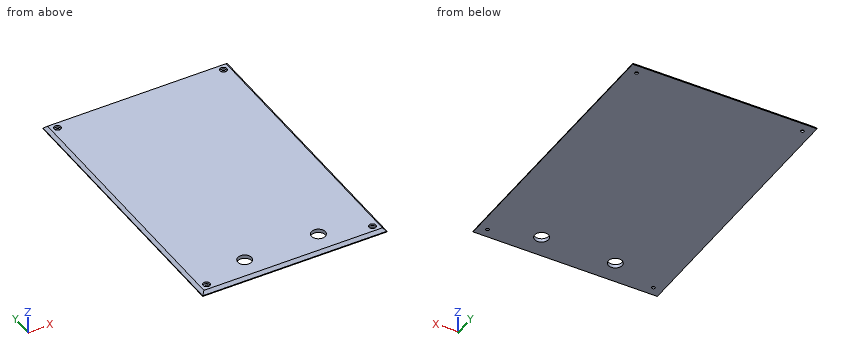
```python
from build123d import *

# Parameters (mm, degrees)
SKETCH1_W                                           = 254
SKETCH1_H                                           = 381
BOSS_EXTRUDE1_DEPTH                                 = 5
CHAMFER1_SIZE                                       = 4
CBORE_FOR_8_BINDING_HEAD_MACHINE_SCREW1_D           = 4.4958
CBORE_FOR_8_BINDING_HEAD_MACHINE_SCREW1_CBORE_D     = 9.525
CBORE_FOR_8_BINDING_HEAD_MACHINE_SCREW1_CBORE_DEPTH = 2.667
LPATTERN1_COUNT                                     = 2
LPATTERN1_PITCH                                     = 355.6
LPATTERN1_COUNT_DIR2                                = 2
LPATTERN1_PITCH_DIR2                                = 228.6
F_19_0_19_DIAMETER_HOLE1_D                          = 19


with BuildPart() as part:
    # Sketch1 → Boss-Extrude1 (new body)
    with BuildSketch(Plane.XY):
        Rectangle(SKETCH1_W, SKETCH1_H)
    extrude(amount=BOSS_EXTRUDE1_DEPTH)

    # Chamfer1
    chamfer1_edges = [part.edges().sort_by_distance(p)[0] for p in [
        (127, 0, 5),
        (0, 190.5, 5),
        (-127, 0, 5),
        (0, -190.5, 5),
    ]]
    chamfer(chamfer1_edges, length=CHAMFER1_SIZE)

    # CBORE for #8 Binding Head Machine Screw1 (through all)
    with Locations(Plane.XY.offset(5)):
        with Locations((-114.3, 177.8)):
            cbore_for_8_binding_head_machine_screw1 = CounterBoreHole(CBORE_FOR_8_BINDING_HEAD_MACHINE_SCREW1_D / 2, CBORE_FOR_8_BINDING_HEAD_MACHINE_SCREW1_CBORE_D / 2, CBORE_FOR_8_BINDING_HEAD_MACHINE_SCREW1_CBORE_DEPTH)

    # LPattern1: CBORE for _8 Binding Head Machine Screw1 2 × 2
    with Locations(*[(j * LPATTERN1_PITCH_DIR2, -i * LPATTERN1_PITCH, 0) for i in range(LPATTERN1_COUNT) for j in range(LPATTERN1_COUNT_DIR2) if (i, j) != (0, 0)]):
        add(cbore_for_8_binding_head_machine_screw1, mode=Mode.SUBTRACT)

    # Ø19.0 (19) Diameter Hole1 (through all)
    with Locations(Plane.XY.offset(5)):
        with Locations((-50.8, -158.75), (50.8, -158.75)):
            Hole(F_19_0_19_DIAMETER_HOLE1_D / 2)


solid = part.part
```
Could you check a few things on this model? Use its own coordinates, in mm. Give positions to 0.01 mm unless a question says otherwise; leave off trailing zeros. Loops run counter-clockwise (first coordinate to the right, second up) from the corner with the lowest first, then second, coordinate; pieces in that order, holes last. Notation, with made-up numbers: (-35.5, 22.25) - (-24.5, 22.25) arc R17 ccw to (-24.5, 42.25) - close; hole circle Ø4 at (39, 22.5). An arc over 180 degrees is marked (long way). Answer in a Markdown table with one row per item. Add a question column.
Q1. If we section it at A-A (x = -50.8): List the corners of the cut face in (y, z) for me, plus the area to 3 significant figures.
Q2. For pin 1 (7 mm diameter, centred on x = 114.3, y = 177.8, fed in from +Z); pin 2 (22 mm diameter, centred on x = 50.8, y = -158.75, fed in from -Z); pin 3 (3 mm diameter, centred on y = 46, z = 3, fed in from -X), each with a flat end and sliding along its axis, tell me the tip position at first contact or that it passes through.
Q3. If we section it at C-C (x = 53): List the corners of the cut face in (y, z) for me.
Q4. Please list where these lines run through material, in increasing order: L1, parallel to X at y = 177.8, z = 0.95; L2, parallel to X at y = -177.8, z = 1.6; L3, parallel to Y at x = -114.3, z = 3.05. Write a range as from..to.
Q5. If we section it at B-B (y = -158.75): List the corners of the cut face in (x, z) for me.
The answers:
| question | item | result |
|---|---|---|
| 1 | outline | (-190.5, 0) - (-168.25, 0) - (-168.25, 5) - (-186.5, 5) - (-190.5, 1) - close; (-149.25, 0) - (190.5, 0) - (190.5, 1) - (186.5, 5) - (-149.25, 5) - close |
| 1 | area | 1,790 mm^2 |
| 2 | pin 1 | stops at z = 2.33 |
| 2 | pin 2 | stops at z = 0 |
| 2 | pin 3 | stops at x = -126.5 |
| 3 | outline | (-190.5, 0) - (-167.99, 0) - (-167.99, 5) - (-186.5, 5) - (-190.5, 1) - close; (-149.51, 0) - (190.5, 0) - (190.5, 1) - (186.5, 5) - (-149.51, 5) - close |
| 4 | L1 | x = -127..-116.55, -112.05..112.05, 116.55..127 |
| 4 | L2 | x = -126.4..-116.55, -112.05..112.05, 116.55..126.4 |
| 4 | L3 | y = -188.45..-182.56, -173.04..173.04, 182.56..188.45 |
| 5 | outline | (-127, 0) - (-60.3, 0) - (-60.3, 5) - (-123, 5) - (-127, 1) - close; (-41.3, 0) - (41.3, 0) - (41.3, 5) - (-41.3, 5) - close; (60.3, 0) - (127, 0) - (127, 1) - (123, 5) - (60.3, 5) - close |
